from build123d import *

# Parameters (mm, degrees)
F0_W     = 85
F0_H     = 52
F1_DEPTH = 3
F2_R     = 1.75
F3_DEPTH = 25
F4_W     = 73
F4_H     = 48
F4_W_2   = 71
F4_H_2   = 46
F5_DEPTH = 4
F6_W     = 4
F6_H     = 1
F7_DEPTH = 4


with BuildPart() as f1:
    # F0 (on Top) → F1 (new body)
    with BuildSketch(Plane.XY):
        Rectangle(F0_W, F0_H)
    extrude(amount=F1_DEPTH)

    # F2 (on face) → F3 (cut)
    with BuildSketch(Plane.XY.offset(3)):
        with Locations((-39.75, 22)):
            Circle(F2_R)
        with Locations((-39.75, -22)):
            Circle(F2_R)
        with Locations((39.75, 22)):
            Circle(F2_R)
        with Locations((39.75, -22)):
            Circle(F2_R)
    extrude(amount=-F3_DEPTH, mode=Mode.SUBTRACT)

    # F4 (on face) → F5 (join)
    with BuildSketch(Plane.XY.offset(3)):
        Rectangle(F4_W, F4_H)
        Rectangle(F4_W_2, F4_H_2, mode=Mode.SUBTRACT)
    extrude(amount=F5_DEPTH)

    # F6 (on face) → F7 (cut)
    with BuildSketch(Plane.XY.offset(7)):
        with Locations((22, -23.5)):
            Rectangle(F6_W, F6_H)
    extrude(amount=-F7_DEPTH, mode=Mode.SUBTRACT)


solid = f1.part
Work out the finished part from the listing and answer in its coordinate system (mm). A direction names the side the tool comes from. Round coordinates to 2 decimals unless told otherwise and drop trailing zeros. Loops run counter-clockwise (first coordinate to the right, second up) from the corner with the lowest first, then second, coordinate; pieces in that order, holes last. Notation, with made-up numbers: (53.5, -18) - (97.5, -18) arc R21 cw to (97.5, 0) - close; hole circle Ø3 at (-11, 71.25). An arc over 180 degrees is marked (long way). Use one line per item in the form item = value. Start each with the question number.
(1) Flat-ended cylindrical pins translate along their axes: P1, Ø5, axis at x = 2.5, y = -1, coming from the +Z side; P2, Ø2, axis at x = 39.75, y = 22, coming from the -Z side; P3, Ø2, axis at x = -20, z = 5.5, coming from the +Y side; P4, Ø0.5, axis at y = -23.5, z = 5.5, coming from the +X side. Find the tip coordinate at first contact, or state that the pin passes through.
(2) Find section B-B on x = -39.75. Determine the outline of the cut face in (y, z), and give its area (3 significant figures).
(3) Find section D-D on y = -1.5. Determine the outline of the cut face in (x, z), and give its area (3 significant figures).
(4) Determine the mould class of faces 1 (the face through (-9, -24, 5)), 2 (the face through (42.5, 0, 1)), 3 (the face through (-38.809, 23.476, 1.521)) for opening direction Y: +Y half, -Y half, draft (parallel to the pull), parting line (faces both ways), or undercut.
(5) Which of the six approach directions +Z, -Z, +X, -X, +Y, -Y give full straight-line access (tool end or side, diameter ignored) to faces 4 (the face through (-8, -23, 5)), 5 (the face through (-1, 24, 5)), 6 (the face through (-36.5, 0, 5)), 7 (the face through (-42.5, 0, 1)), 8 (the face through (-1, 0, 0))?
(6) Find section A-A on y = 22. Determine the outline of the cut face in (x, z), and give its area (3 significant figures).
(7) Consider line 1 (Y direction, x = 39.75, z = 1.9); line 2 (X direction, y = -16, z = 3.25); line 3 (Y direction, x = 4, z = 3.25). Determine where each line is inside the solid, lowest interval first.
(8) Find section C-C on z = 4. Determine the outline of the cut face in (x, y), and give its area (3 significant figures).
Answer list:
q1.P1 = 3
q1.P2 = through
q1.P3 = 24
q1.P4 = 36.5
q2.outline = (-26, 0) - (-23.75, 0) - (-23.75, 3) - (-26, 3) - close; (-20.25, 0) - (20.25, 0) - (20.25, 3) - (-20.25, 3) - close; (23.75, 0) - (26, 0) - (26, 3) - (23.75, 3) - close
q2.area = 135 mm^2
q3.outline = (-42.5, 0) - (42.5, 0) - (42.5, 3) - (36.5, 3) - (36.5, 7) - (35.5, 7) - (35.5, 3) - (-35.5, 3) - (-35.5, 7) - (-36.5, 7) - (-36.5, 3) - (-42.5, 3) - close
q3.area = 263 mm^2
q4.face_1 = -Y half
q4.face_2 = draft
q4.face_3 = undercut
q5.face_4 = +Z
q5.face_5 = +Z, +X, -X, +Y
q5.face_6 = +Z, -X, +Y, -Y
q5.face_7 = +Z, -Z, -X, +Y, -Y
q5.face_8 = -Z, +X, -X, +Y, -Y
q6.outline = (-42.5, 0) - (-41.5, 0) - (-41.5, 3) - (-42.5, 3) - close; (-38, 0) - (38, 0) - (38, 3) - (36.5, 3) - (36.5, 7) - (35.5, 7) - (35.5, 3) - (-35.5, 3) - (-35.5, 7) - (-36.5, 7) - (-36.5, 3) - (-38, 3) - close; (41.5, 0) - (42.5, 0) - (42.5, 3) - (41.5, 3) - close
q6.area = 242 mm^2
q7.line_1 = -26 to -23.75, -20.25 to 20.25, 23.75 to 26
q7.line_2 = -36.5 to -35.5, 35.5 to 36.5
q7.line_3 = -24 to -23, 23 to 24
q8.outline = (-36.5, -24) - (20, -24) - (20, -23) - (-35.5, -23) - (-35.5, 23) - (35.5, 23) - (35.5, -23) - (24, -23) - (24, -24) - (36.5, -24) - (36.5, 24) - (-36.5, 24) - close
q8.area = 234 mm^2
